Verification items for the finished model (mm, model axes). Face numbers are marked on the shaded views. A direction names the side the tool comes from. Coordinates: 2 decimals unless noted, no trailing zeros. Write each loop counter-clockwise with the first axis right and the second up, starting at its lowest first coordinate (ties: lowest second). Pieces come first, ordered by that corner, then holes. Notation, with made-up numbers: (74.25, 61.5) -> (118.25, 61.5) arc R20 cw to (118.25, 94.5) -> close; hole circle Ø2 at (-32, 0). An arc over 180 degrees is marked (long way). Write item = value, one per line. Start each with the question number.
(1) Set-up check for the marked faces 1 and 2: record each of +Z, -Z, +X, -X, +Y, -Y from which the full face is reachable in a straight line by a thin tool's end or side.
(2) Material ranges on probe 1 along Y at (x, z) = (-42, 1.75); probe 2 along Y at (x, z) = (7.5, 6.5); probe 3 along X at (y, z) = (16, 15), recorded low to high. Write a range as [from, to].
(3) Section check D-D (x = 35.5). Record the cut outline in (y, z).
(4) Section check A-A (x = 0). Record the cut outline in (y, z).
(5) Section check C-C (z = 10). Record the cut outline in (x, y), plus the area to 3 significant figures.
(6) Gauge pin test, flat ends, axial feed: pin 1 Ø6 at (x, z) = (-21, 8) entering from -Y; pin 2 Ø6 at (y, z) = (0.5, 12.5) entering from -X; pin 3 Ø1.5 at (y, z) = (-1, 11) entering from +X. Record the tip position at first contact, or that the pin passes through.
(7) Section check B-B (y = 16.5). Record the cut outline in (x, z), plus the area to 3 significant figures.
Autodesk Inventor part; units mm, degrees
ref_plane "YZ Plane" through (0, 0, 0) normal (1, 0, 0) x (0, 1, 0)
ref_plane "XZ Plane" through (0, 0, 0) normal (0, 1, 0) x (-1, 0, 0)
ref_plane "XY Plane" through (0, 0, 0) normal (0, 0, 1) x (1, 0, 0)
sketch "Sketch1" plane through (0, 0, 0) normal (0, 0, 1) x (1, 0, 0)
  line L0 (-50, 20) -> (50, 20)
  line L1 (-50, 20) -> (-50, 13.65)
  line L2 (-50, 13.65) -> (50, 13.65)
  line L3 (50, 13.65) -> (50, 20)
  line L4 (54, 24) -> (-54, 24)
  line L5 (-54, 24) -> (-54, 9.65)
  line L6 (-54, 9.65) -> (54, 9.65)
  line L7 (54, 9.65) -> (54, 24)
  point P0 (0, 0)
  dimension "d0" = 100
  dimension "d1" = 6.35
  dimension "d2" = 4
extrude "Extrusion1" add sketch "Sketch1" along normal blind 20
sketch "Sketch2" plane through (-54, 9.65, 0) normal (0, -1, 0) x (1, 0, 0)
  circle A0 centre (54, 10) radius 6
  point P0 (54, 0)
  dimension "d5" = 12
extrude "Extrusion2" add sketch "Sketch2" along normal blind 20
sketch "Sketch3" plane through (-54, 9.65, 0) normal (0, -1, 0) x (1, 0, 0)
  circle A0 centre (54, 10) radius 6
  circle A1 centre (54, 10) radius 8.5725
  point P0 (54, 0)
  dimension "d8" = 17.145
extrude "Extrusion3" add sketch "Sketch3" along normal blind 14.4
properties part number "Bracket"
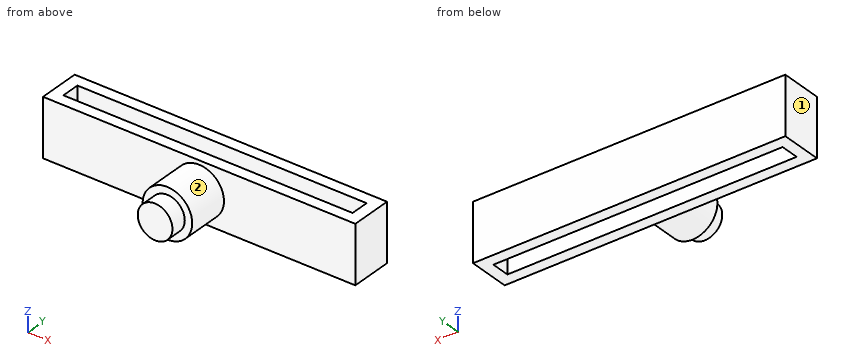
Response:
q1.face_1 = +Z, -Z, -X, +Y, -Y
q1.face_2 = -Y
q2.probe_1 = [9.65, 13.65], [20, 24]
q2.probe_2 = [-4.75, 13.65], [20, 24]
q2.probe_3 = [-54, -50], [50, 54]
q3.outline = (9.65, 0) -> (13.65, 0) -> (13.65, 20) -> (9.65, 20) -> close; (20, 0) -> (24, 0) -> (24, 20) -> (20, 20) -> close
q4.outline = (-10.35, 4) -> (-4.75, 4) -> (-4.75, 1.43) -> (9.65, 1.43) -> (9.65, 0) -> (13.65, 0) -> (13.65, 20) -> (9.65, 20) -> (9.65, 18.57) -> (-4.75, 18.57) -> (-4.75, 16) -> (-10.35, 16) -> close; (20, 0) -> (24, 0) -> (24, 20) -> (20, 20) -> close
q5.outline = (-54, 9.65) -> (-8.57, 9.65) -> (-8.57, -4.75) -> (-6, -4.75) -> (-6, -10.35) -> (6, -10.35) -> (6, -4.75) -> (8.57, -4.75) -> (8.57, 9.65) -> (54, 9.65) -> (54, 24) -> (-54, 24) -> close; hole (-50, 13.65) -> (50, 13.65) -> (50, 20) -> (-50, 20) -> close
q5.area = 1,230 mm2
q6.pin_1 = 9.65
q6.pin_2 = -8.57
q6.pin_3 = 8.57
q7.outline = (-54, 0) -> (-50, 0) -> (-50, 20) -> (-54, 20) -> close; (50, 0) -> (54, 0) -> (54, 20) -> (50, 20) -> close
q7.area = 160 mm2
